Part model, mm, in its own coordinate system. A direction names the side the tool comes from. Round coordinates to 2 decimals unless told otherwise and drop trailing zeros. Write each loop counter-clockwise with the first axis right and the second up, starting at its lowest first coordinate (ties: lowest second). Pieces come first, ordered by that corner, then holes. Notation, with made-up numbers: M -32,-21.75 L -23,-21.75 A9 ccw -23,-4.75 Z; hole C 50.25,64.25 d4. An arc over 180 degrees is marked long. Use a Markdown table: item, result. Add a question column.
1) Slice it at B-B on y = 8. Write the cut outline in (x, z).
2) Drop flat-ended pins along their axis: P1, Ø1, axis at y = -5, z = 5.5, coming from the -X side; P2, Ø6.5, axis at x = -15.5, y = 82, coming from the +Z side; P3, Ø3.5, axis at x = -1, y = -1, coming from the +Z side. Give the stop position or say it passes through.
3) Which spindle directions (+Z, -Z, +X, -X, +Y, -Y) get a long thin tool onto all of the face, cutting with end or side? Do faces 5 (the face through (0, 26, -11)), 6 (the face through (-15, 83, -9)), 7 (the face through (15, 79.452, -5)), 8 (the face through (-15, 79.452, -5)). Say none if no direction does.
4) Two-plate mould, pull along X, no slides. Class faces 1 (the face through (0, -3.5, 7)), 2 (the face through (12.7, 55.07, -5.42)), 3 (the face through (15, 86.452, -5)), 4 (the face through (0, 0, -6)): released by +X, released by -X, zero draft, split by the parting line, or undercut.
5) Slice it at A-A on z = 8.25. Write the cut outline in (x, y).
6) Slice it at D-D on y = 22.5. Write the cut outline in (x, z), plus the area to 3 significant figures.
7) Slice it at C-C on x = 21.5. Write the cut outline in (y, z), plus the area to 3 significant figures.
8) Wall check: probe 1 along Y at (x, z) = (0, -7.65); probe 2 along Z at (x, y) = (20, 18); probe 3 along X at (y, z) = (82, -12.75). Give the ranges that are in metal, low to high.
```python
from build123d import *

# Parameters (mm, degrees)
SKETCH1_R                = 20
SKETCH1_R_2              = 4
BOSS_EXTRUDE1_DEPTH      = 11
SKETCH1_4_R              = 20
BOSS_EXTRUDE2_DEPTH      = 6
SKETCH3_R                = 16
BOSS_EXTRUDE3_DEPTH      = 10
SKETCH4_W                = 7
SKETCH4_H                = 7
CUT_EXTRUDE1_DEPTH       = 7
BOSS_EXTRUDE4_DEPTH      = 7
BOSS_EXTRUDE4_DEPTH_BACK = 18
SKETCH5_W                = 25
SKETCH5_H                = 25
SKETCH6_W                = 7
SKETCH6_H                = 7
BOSS_EXTRUDE5_DEPTH      = 6
CUT_EXTRUDE2_DEPTH       = 11
FILLET1_R                = 7
FILLET2_R                = 7
FILLET3_R                = 8


with BuildPart() as part:
    # Sketch1 → Boss-Extrude1 (new body)
    with BuildSketch(Plane.XY):
        with BuildLine():
            Line((-27.617597302, -2.366025969), (-13.325344527, 51.86810446))
            ThreePointArc((-13.325344527, 51.86810446), (-12.707194725, 55.026842667), (-12.5, 58.238821277))
            Line((-12.5, 58.238821277), (-12.5, 67.307346))
            Line((-12.5, 67.307346), (-12.5, 95.903667694))
            ThreePointArc((-12.5, 95.903667694), (0, 100.951833847), (12.5, 95.903667694))
            Line((12.5, 95.903667694), (12.5, 67.307346))
            Line((12.5, 67.307346), (12.5, 58.238821277))
            ThreePointArc((12.5, 58.238821277), (12.707194725, 55.026842667), (13.325344527, 51.86810446))
            Line((13.325344527, 51.86810446), (27.617597302, -2.366025969))
            ThreePointArc((27.617597302, -2.366025969), (25.744947954, -20.033668156), (12.608807935, -31.995867846))
            ThreePointArc((12.608807935, -31.995867846), (0, -34.390661476), (-12.608807935, -31.995867846))
            ThreePointArc((-12.608807935, -31.995867846), (-25.744947954, -20.033668156), (-27.617597302, -2.366025969))
        make_face()
        Circle(SKETCH1_R, mode=Mode.SUBTRACT)
        with Locations((0, 82.951833847)):
            Circle(SKETCH1_R_2, mode=Mode.SUBTRACT)
    extrude(amount=-BOSS_EXTRUDE1_DEPTH)

    # Sketch1<4> → Boss-Extrude2 (add)
    with BuildSketch(Plane.XY):
        Circle(SKETCH1_4_R)
    extrude(amount=-BOSS_EXTRUDE2_DEPTH)

    # Sketch3 → Boss-Extrude3 (add)
    with BuildSketch(Plane.XY):
        Circle(SKETCH3_R)
    extrude(amount=BOSS_EXTRUDE3_DEPTH)

    # Sketch4 → Cut-Extrude1 (cut)
    with BuildSketch(Plane.XY.offset(10)):
        Rectangle(SKETCH4_W, SKETCH4_H)
    extrude(amount=-CUT_EXTRUDE1_DEPTH, mode=Mode.SUBTRACT)

    # Sketch5 → Boss-Extrude4 (add, two sides: drawn at the far end of the back side and taken through both)
    with BuildSketch(Plane.XY.offset(-BOSS_EXTRUDE4_DEPTH_BACK)):
        with Locations((0, 82.951833847)):
            Rectangle(SKETCH5_W, SKETCH5_H)
    extrude(amount=BOSS_EXTRUDE4_DEPTH + BOSS_EXTRUDE4_DEPTH_BACK)

    # Sketch6 → Boss-Extrude5 (add)
    with BuildSketch(Plane(origin=(12.5, 0, 0), x_dir=(0, 0, -1), z_dir=(1, 0, 0))):
        with Locations((5.5, 82.951833847)):
            Rectangle(SKETCH6_W, SKETCH6_H)
    boss_extrude5 = extrude(amount=BOSS_EXTRUDE5_DEPTH)

    # Mirror1: Boss-Extrude5 across plane
    add(boss_extrude5.mirror(Plane(origin=(0, 0, 0), x_dir=(0, 0, 1), z_dir=(1, 0, 0))))

    # Sketch7 → Cut-Extrude2 (cut)
    with BuildSketch(Plane.XY):
        with BuildLine():
            Line((-12.5, 95.451833847), (12.5, 95.451833847))
            Line((12.5, 95.451833847), (12.5, 95.903667694))
            ThreePointArc((12.5, 95.903667694), (0, 100.951833847), (-12.5, 95.903667694))
            Line((-12.5, 95.903667694), (-12.5, 95.451833847))
        make_face()
    extrude(amount=-CUT_EXTRUDE2_DEPTH, mode=Mode.SUBTRACT)

    # Fillet1
    fillet1_edges = [part.edges().sort_by_distance(p)[0] for p in [
        (0, 70.451833847, 0),
    ]]
    fillet(fillet1_edges, radius=FILLET1_R - 0.0001)  # a hair under: the kernel refuses the full size

    # Fillet2
    fillet2_edges = [part.edges().sort_by_distance(p)[0] for p in [
        (0, 70.451833847, -11),
    ]]
    fillet(fillet2_edges, radius=FILLET2_R - 0.0001)  # a hair under: the kernel refuses the full size

    # Fillet3
    fillet3_edges = [part.edges().sort_by_distance(p)[0] for p in [
        (0, 70.451833847, -18),
        (0, 95.451833847, -18),
        (0, 95.451833847, 7),
        (0, 70.451833847, 7),
    ]]
    fillet(fillet3_edges, radius=FILLET3_R)


solid = part.part
```
Entries:
| question | item | result |
|---|---|---|
| 1 | outline | M -24.89,-11 L -18.33,-11 L -18.33,-6 L 18.33,-6 L 18.33,-11 L 24.89,-11 L 24.89,0 L 13.86,0 L 13.86,10 L -13.86,10 L -13.86,0 L -24.89,0 Z |
| 2 | P1 | stops at x = -15.35 |
| 2 | P2 | stops at z = 7 |
| 2 | P3 | stops at z = 3 |
| 3 | face 5 | -Z, +X, -X, -Y |
| 3 | face 6 | -Z, -X, +Y |
| 3 | face 7 | +Z, -Z, +X |
| 3 | face 8 | +Z, -Z, -X |
| 4 | face 1 | undercut |
| 4 | face 2 | released by +X |
| 4 | face 3 | zero draft |
| 4 | face 4 | undercut |
| 5 | outline | C 0,0 d32; hole M -3.5,-3.5 L 3.5,-3.5 L 3.5,3.5 L -3.5,3.5 Z |
| 6 | outline | M -21.06,-11 L 21.06,-11 L 21.06,0 L -21.06,0 Z |
| 6 | area | 463 mm^2 |
| 7 | outline | M -26.03,-11 L 20.85,-11 L 20.85,0 L -26.03,0 Z |
| 7 | area | 516 mm^2 |
| 8 | probe 1 | y = -34.39 to -20, 20 to 95.45 |
| 8 | probe 2 | z = -11 to 0 |
| 8 | probe 3 | x = -12.5 to 12.5 |
